Autodesk Inventor part; units mm, degrees
ref_plane "YZ Plane" through (0, 0, 0) normal (1, 0, 0) x (0, 1, 0)
ref_plane "XZ Plane" through (0, 0, 0) normal (0, 1, 0) x (-1, 0, 0)
ref_plane "XY Plane" through (0, 0, 0) normal (0, 0, 1) x (1, 0, 0)
sketch "Sketch1" plane through (0, 0, 0) normal (0, 0, 1) x (1, 0, 0)
  line L0 (-46.8, 0) -> (62.4, 0)
  line L1 (0, 7.8) -> (0, -0.6)
  line L2 (-39, 0) -> (-39, 4)
  line L3 (-39, 4) -> (-30.0485, 4)
  line L4 (-30.0485, 4) -> (-29.5, 3.05)
  line L5 (-29.5, 3.05) -> (-27, 3.05)
  line L6 (-27, 3.05) -> (-27, 6)
  line L7 (-27, 6) -> (27, 6)
  line L8 (27, 6) -> (27, 3.05)
  line L9 (27, 3.05) -> (29.5, 3.05)
  line L10 (29.5, 3.05) -> (30.0485, 4)
  line L11 (30.0485, 4) -> (39, 4)
  line L12 (39, 4) -> (39, 0)
  line L13 (-39, 0) -> (39, 0)
  dimension "d0" = 4
  dimension "d1" = 60
  dimension "d2" = 12
  dimension "d3" = 78
  dimension "d4" = 3.05
  dimension "d5" = 60
  dimension "d6" = 4
  dimension "d7" = 12
  dimension "d8" = 6
  dimension "d9" = 2.5
  dimension "d10" = 2.5
  dimension "d11" = 3.05
revolve "Revolution1" add sketch "Sketch1" angle 360 about axis through (-39, 0, 0) along (1, 0, 0)
chamfer "Chamfer1" distance 1 angle 45 2 edges at (39, -4, 0) (-39, -4, 0)
fillet "Fillet1" radius 0.6 2 edges at (-27, -3.05, 0) (27, -3.05, 0)
properties part number "Pin Seized"
Geometry: final body of the model. Coordinates: model frame, mm. A direction names the side the tool comes from. Give positions to 0.01 mm unless a question says otherwise; leave off trailing zeros. Write each loop counter-clockwise with the first axis right and the second up, starting at its lowest first coordinate (ties: lowest second). Pieces come first, ordered by that corner, then holes. Notation, with made-up numbers: (49, 72.5) -> (79, 72.5) arc R26 cw to (79, 90.5) -> close; hole circle Ø9 at (-22, 30.25). An arc over 180 degrees is marked (long way). Answer as a JSON object with one key per item and string values.
1. Cut plane C-C on x = 15.5. Output: boundary loops of the cut face in (y, z), and give its area (3 significant figures).
Ans:
{"outline": "circle Ø12 at (0, 0)", "area": "113 mm^2"}
2. Contact query for flat-ended pins moving along their axis: pin 1 (5 mm diameter, centred on x = 19.5, y = 1, fed in from +Z); pin 2 (1.5 mm diameter, centred on x = 25.5, y = 3, fed in from -Z); pin 3 (1 mm diameter, centred on x = 5, z = -1, fed in from -Y). Output: stop coordinate, or through.
Ans:
{"pin 1": "stops at z = 6", "pin 2": "stops at z = -5.56", "pin 3": "stops at y = -5.98"}
3. Cut plane A-A on z = 0. Output: boundary loops of the cut face in (x, y), and give its area (3 significant figures).
Ans:
{"outline": "(-39, -3) -> (-38, -4) -> (-30.05, -4) -> (-29.5, -3.05) -> (-27.6, -3.05) arc R0.6 cw to (-27, -3.65) -> (-27, -6) -> (27, -6) -> (27, -3.65) arc R0.6 cw to (27.6, -3.05) -> (29.5, -3.05) -> (30.05, -4) -> (38, -4) -> (39, -3) -> (39, 3) -> (38, 4) -> (30.05, 4) -> (29.5, 3.05) -> (27.6, 3.05) arc R0.6 cw to (27, 3.65) -> (27, 6) -> (-27, 6) -> (-27, 3.65) arc R0.6 cw to (-27.6, 3.05) -> (-29.5, 3.05) -> (-30.05, 4) -> (-38, 4) -> (-39, 3) -> close", "area": "828 mm^2"}
4. Ray query, probe 1 along X at (y, z) = (-2.5, -2); probe 2 along Y at (x, z) = (-14, 4.75); probe 3 along X at (y, z) = (-3.5, -4.25). Return the intervals inside material, ascending. Write a range as from..to.
Ans:
{"probe 1": "x = -38.8..-29.59, -27.2..27.2, 29.59..38.8", "probe 2": "y = -3.67..3.67", "probe 3": "x = -27..27"}
5. Access query for faces 4 (the cylindrical face through (0, -6, 0)), 5 (the cylindrical face through (34.08, -0.867, -3.905)), 6 (the flat face through (27, 3, -3)), 7 (the cylindrical face through (-33.969, -0.867, -3.905)). Directions: +Z, -Z, +X, -X, +Y, -Y. A direction counts if a zero-diameter tool reaches every point of the face in a straight line with its end or side. Return the directions, or none.
Ans:
{"face 4": "+X, -X", "face 5": "+X", "face 6": "none", "face 7": "-X"}
6. Cut plane D-D on y = 4.75. Output: boundary loops of the cut face in (x, z).
Ans:
{"outline": "(-27, -3.67) -> (27, -3.67) -> (27, 3.67) -> (-27, 3.67) -> close"}
7. Mould query, pull axis X, two halves, no side actions, for faces 1 (the flat face through (-39, 0, 0)), 2 (the flat face through (39, 0, 0)), 3 (the cylindrical face through (28.563, -3.047, 0.134)). Classes: pulls with the +X half, pulls with the -X half, needs draft (parallel to the pull), parting line crosses it, or undercut.
Ans:
{"face 1": "pulls with the -X half", "face 2": "pulls with the +X half", "face 3": "undercut"}
